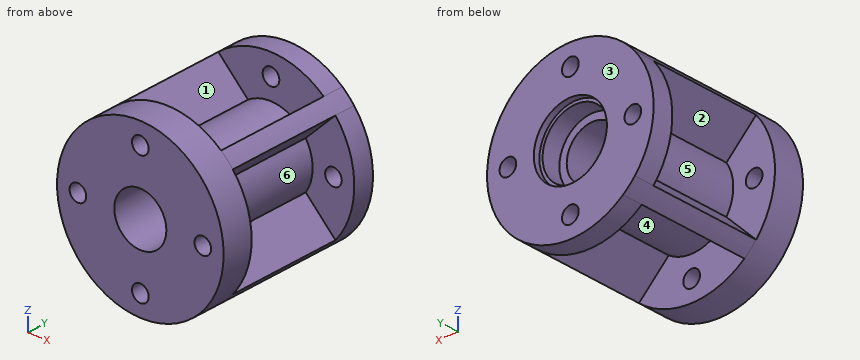
```python
from build123d import *

# Parameters (mm, degrees)
SKETCH1_R           = 40
SKETCH1_R_2         = 12.5
BOSS_EXTRUDE1_DEPTH = 15
SKETCH3_R           = 20
SKETCH3_R_2         = 12.5
BOSS_EXTRUDE2_DEPTH = 53
SKETCH4_R           = 20
SKETCH4_R_2         = 16.05
BOSS_EXTRUDE3_DEPTH = 12
BOSS_EXTRUDE4_DEPTH = 65
SKETCH6_R           = 17.55
CUT_EXTRUDE2_DEPTH  = 3
SKETCH7_R           = 40
SKETCH7_R_2         = 20
BOSS_EXTRUDE5_DEPTH = 10
SKETCH2_R           = 4
CUT_EXTRUDE1_DEPTH  = 80


with BuildPart() as part:
    # Sketch1 → Boss-Extrude1 (new body)
    with BuildSketch(Plane(origin=(0, 0, 0), x_dir=(1, 0, 0), z_dir=(0, 1, 0))):
        Circle(SKETCH1_R)
        Circle(SKETCH1_R_2, mode=Mode.SUBTRACT)
    extrude(amount=BOSS_EXTRUDE1_DEPTH)

    # Sketch3 → Boss-Extrude2 (add)
    with BuildSketch(Plane(origin=(0, 15, 0), x_dir=(1, 0, 0), z_dir=(0, 1, 0))):
        Circle(SKETCH3_R)
        Circle(SKETCH3_R_2, mode=Mode.SUBTRACT)
    extrude(amount=BOSS_EXTRUDE2_DEPTH)

    # Sketch4 → Boss-Extrude3 (add)
    with BuildSketch(Plane(origin=(0, 68, 0), x_dir=(1, 0, 0), z_dir=(0, 1, 0))):
        Circle(SKETCH4_R)
        Circle(SKETCH4_R_2, mode=Mode.SUBTRACT)
    extrude(amount=BOSS_EXTRUDE3_DEPTH)

    # Sketch5 → Boss-Extrude4 (add)
    with BuildSketch(Plane(origin=(0, 15, 0), x_dir=(1, 0, 0), z_dir=(0, 1, 0))):
        with BuildLine():
            Line((-16.684833585, -11.027979336), (-30.970921684, -25.314067434))
            ThreePointArc((-30.970921684, -25.314067434), (-28.284271247, -28.284271247), (-25.314067434, -30.970921684))
            Line((-25.314067434, -30.970921684), (-11.027979336, -16.684833585))
            ThreePointArc((-11.027979336, -16.684833585), (-14.142135624, -14.142135624), (-16.684833585, -11.027979336))
        make_face()
        with BuildLine():
            Line((-16.684833585, 11.027979336), (-30.970921684, 25.314067434))
            ThreePointArc((-30.970921684, 25.314067434), (-28.284271247, 28.284271247), (-25.314067434, 30.970921684))
            Line((-25.314067434, 30.970921684), (-11.027979336, 16.684833585))
            ThreePointArc((-11.027979336, 16.684833585), (-14.142135624, 14.142135624), (-16.684833585, 11.027979336))
        make_face()
        with BuildLine():
            Line((11.027979336, 16.684833585), (25.314067434, 30.970921684))
            ThreePointArc((25.314067434, 30.970921684), (28.284271247, 28.284271247), (30.970921684, 25.314067434))
            Line((30.970921684, 25.314067434), (16.684833585, 11.027979336))
            ThreePointArc((16.684833585, 11.027979336), (14.142135624, 14.142135624), (11.027979336, 16.684833585))
        make_face()
        with BuildLine():
            Line((16.684833585, -11.027979336), (30.970921684, -25.314067434))
            ThreePointArc((30.970921684, -25.314067434), (28.284271247, -28.284271247), (25.314067434, -30.970921684))
            Line((25.314067434, -30.970921684), (11.027979336, -16.684833585))
            ThreePointArc((11.027979336, -16.684833585), (14.142135624, -14.142135624), (16.684833585, -11.027979336))
        make_face()
    extrude(amount=BOSS_EXTRUDE4_DEPTH)

    # Sketch6 → Cut-Extrude2 (cut)
    with BuildSketch(Plane(origin=(0, 80, 0), x_dir=(1, 0, 0), z_dir=(0, 1, 0))):
        Circle(SKETCH6_R)
    extrude(amount=-CUT_EXTRUDE2_DEPTH, mode=Mode.SUBTRACT)

    # Sketch7 → Boss-Extrude5 (add)
    with BuildSketch(Plane(origin=(0, 80, 0), x_dir=(1, 0, 0), z_dir=(0, 1, 0))):
        Circle(SKETCH7_R)
        Circle(SKETCH7_R_2, mode=Mode.SUBTRACT)
    extrude(amount=-BOSS_EXTRUDE5_DEPTH)

    # Sketch2 → Cut-Extrude1 (cut)
    with BuildSketch(Plane(origin=(0, 0, 0), x_dir=(1, 0, 0), z_dir=(0, 1, 0))):
        with Locations((0, 30)):
            Circle(SKETCH2_R)
        with Locations((30, 0)):
            Circle(SKETCH2_R)
        with Locations((0, -30)):
            Circle(SKETCH2_R)
        with Locations((-30, 0)):
            Circle(SKETCH2_R)
    extrude(amount=CUT_EXTRUDE1_DEPTH, mode=Mode.SUBTRACT)


solid = part.part
```
Geometry check sheet. Reference: the model listing, model coordinates, mm. Face numbers are marked on the shaded views. A direction names the side the tool comes from. Round coordinates to 2 decimals unless told otherwise and drop trailing zeros. Order: outer loops, then holes, each group sorted by start corner. A loop starts at its lowest first (then second) coordinate and runs counter-clockwise, first axis right, second up. Notation, with made-up numbers: (75.25, -28.75) - (92.25, -28.75) arc R34 cw to (92.25, 1.25) - close; hole circle Ø2 at (12.25, 73.5). An arc over 180 degrees is marked (long way). Use a Markdown table: item, result. Add a question column.
(1) Sectioned sample at A-A, the plane y = 35. Enter the section's corners in (x, z).
(2) Sectioned sample at D-D, the plane y = 13. Enter the section's corners in (x, z), and give its area (3 significant figures).
(3) Sectioned sample at C-C, the plane z = 8.5. Enter the section's corners in (x, y), and give its area (3 significant figures).
(4) Sectioned sample at B-B, the plane x = 7.5. Enter the section's corners in (y, z), and give its area (3 significant figures).
(5) Depth check by flat-ended pin: pin 1 (10 mm diameter, centred on x = -11, y = 33, fed in from -Z); pin 2 (5 mm diameter, centred on y = 46, z = -1.5, fed in from -X); pin 3 (6 mm diameter, centred on y = 41.5, z = 8.5, fed in from -X). Enter the tip coordinate at first touch or a pass-through.
(6) Tool access check on the marked faces 4, 5 and 6. Record the directions out of +Z, -Z, +X, -X, +Y, -Y that give a thin tool (end or side, any length) a straight path to the whole face; none if there is none.
(7) Release check for a two-part mould opening along Z. For the marked faces 1, 2 and 3 record: pulls with the +Z half, pulls with the -Z half, needs draft (parallel to the pull), parting line crosses it, or undercut.
(8) Material ranges on line 1 along X through (y, z) = (78.4, 0); line 2 along Z through (x, y) = (0, 5.75), recorded low to high. Write a range as [from, to].
Answers below:
| question | item | result |
|---|---|---|
| 1 | outline | (-30.97, -25.31) arc R40 ccw to (-25.31, -30.97) - (-11.03, -16.68) arc R20 ccw to (11.03, -16.68) - (25.31, -30.97) arc R40 ccw to (30.97, -25.31) - (16.68, -11.03) arc R20 ccw to (16.68, 11.03) - (30.97, 25.31) arc R40 ccw to (25.31, 30.97) - (11.03, 16.68) arc R20 ccw to (-11.03, 16.68) - (-25.31, 30.97) arc R40 ccw to (-30.97, 25.31) - (-16.68, 11.03) arc R20 ccw to (-16.68, -11.03) - close; hole circle Ø25 at (0, 0) |
| 2 | outline | circle Ø80 at (0, 0); hole circle Ø8 at (-30, 0); hole circle Ø25 at (0, 0); hole circle Ø8 at (0, -30); hole circle Ø8 at (0, 30); hole circle Ø8 at (30, 0) |
| 2 | area | 4,330 mm² |
| 3 | outline | (-39.09, 0) - (-9.17, 0) - (-9.17, 68) - (-13.61, 68) - (-13.61, 77) - (-15.35, 77) - (-15.35, 80) - (-39.09, 80) - (-39.09, 70) - (-18.1, 70) - (-18.1, 15) - (-39.09, 15) - close; (9.17, 0) - (39.09, 0) - (39.09, 15) - (18.1, 15) - (18.1, 70) - (39.09, 70) - (39.09, 80) - (15.35, 80) - (15.35, 77) - (13.61, 77) - (13.61, 68) - (9.17, 68) - close |
| 3 | area | 2,360 mm² |
| 4 | outline | (0, -39.29) - (15, -39.29) - (15, -18.54) - (70, -18.54) - (70, -39.29) - (80, -39.29) - (80, -15.87) - (77, -15.87) - (77, -14.19) - (68, -14.19) - (68, -10) - (0, -10) - close; (0, 10) - (68, 10) - (68, 14.19) - (77, 14.19) - (77, 15.87) - (80, 15.87) - (80, 39.29) - (70, 39.29) - (70, 18.54) - (15, 18.54) - (15, 39.29) - (0, 39.29) - close |
| 4 | area | 2,290 mm² |
| 5 | pin 1 | z = -21.66 |
| 5 | pin 2 | x = -20 |
| 5 | pin 3 | x = -19.23 |
| 6 | face 4 | -Z |
| 6 | face 5 | -X |
| 6 | face 6 | +X |
| 7 | face 1 | pulls with the +Z half |
| 7 | face 2 | undercut |
| 7 | face 3 | needs draft |
| 8 | line 1 | [-40, -34], [-26, -17.55], [17.55, 26], [34, 40] |
| 8 | line 2 | [-40, -34], [-26, -12.5], [12.5, 26], [34, 40] |
